Model file for the job. Use its own axes, mm. Give positions to 0.01 mm unless a question says otherwise; leave off trailing zeros. Loops run counter-clockwise (first coordinate to the right, second up) from the corner with the lowest first, then second, coordinate; pieces in that order, holes last. Notation, with made-up numbers: M 0,2 L 18,2 A12 cw 18,6 Z; hole C -38.75,-15.75 d11. An arc over 180 degrees is marked long. Answer in a Markdown table with one row per item.
```python
from build123d import *

# Parameters (mm, degrees)
SKETCH_1_W          = 46
SKETCH_1_H          = 54
EXTRUDE_1_DEPTH     = 4
SKETCH_5_R          = 1.525
CUT_EXTRUDE_1_DEPTH = 54
FILLET_1_R          = 2


with BuildPart() as part:
    # 草图1 → 凸台-拉伸1 (new body)
    with BuildSketch(Plane.XY):
        Rectangle(SKETCH_1_W, SKETCH_1_H)
    extrude(amount=EXTRUDE_1_DEPTH)

    # 草图5 → 切除-拉伸1 (cut)
    with BuildSketch(Plane(origin=(0, 0, 0), x_dir=(-1, 0, 0), z_dir=(0, 0, -1))):
        with Locations((5, -24)):
            Circle(SKETCH_5_R)
        with Locations((-15, -24)):
            Circle(SKETCH_5_R)
        with Locations((-19, 5.310310448)):
            Circle(SKETCH_5_R)
        with Locations((19, 5.310310448)):
            Circle(SKETCH_5_R)
    extrude(amount=-CUT_EXTRUDE_1_DEPTH, mode=Mode.SUBTRACT)

    # 圆角1
    fillet_1_edges = [part.edges().sort_by_distance(p)[0] for p in [
        (23, -27, 2),
        (-23, -27, 2),
        (-23, 27, 2),
        (23, 27, 2),
    ]]
    fillet(fillet_1_edges, radius=FILLET_1_R)


solid = part.part
```
(1) Wall check: L1, parallel to Y at x = 15, z = 1 (3 decimals); L2, parallel to Y at x = -19, z = 2.1; L3, parallel to X at y = 4.5, z = 1.8. Give the ranges that are in metal, low to high.
Established:
| item | result |
|---|---|
| L1 | y = -27 to -25.525, -22.475 to 27 |
| L2 | y = -27 to 3.79, 6.84 to 27 |
| L3 | x = -23 to -20.29, -17.71 to 17.71, 20.29 to 23 |
(2) Saw through at A-A, the plane y = -24. Give the cut face in (x, z) (3 decimals).
Established:
| item | result |
|---|---|
| outline | M -23,0 L -6.525,0 L -6.525,4 L -23,4 Z; M -3.475,0 L 13.475,0 L 13.475,4 L -3.475,4 Z; M 16.525,0 L 23,0 L 23,4 L 16.525,4 Z |
(3) Saw through at B-B, the plane x = 15. Give the cut face in (y, z) (3 decimals), and give its area (3 significant figures).
Established:
| item | result |
|---|---|
| outline | M -27,0 L -25.525,0 L -25.525,4 L -27,4 Z; M -22.475,0 L 27,0 L 27,4 L -22.475,4 Z |
| area | 204 mm2 |
(4) Flat gauge pin, fed straight in: P1, Ø1.8, axis at x = 15, y = -24, coming from the +Z side. Where does the tip first touch, or does it go through?
Established:
| item | result |
|---|---|
| P1 | passes through |
(5) Mould opens along Y. For faces 1 (the cylindrical face through (22.4, 26.43, 2.03)), 2 (the cylindrical face through (14.296, -25.353, 1.972)), 3 (the flat face through (0, 0, 4)) say: pulls with the +Y half, pulls with the -Y half, needs draft (parallel to the pull), parting line crosses it, or undercut.
Established:
| item | result |
|---|---|
| face 1 | pulls with the +Y half |
| face 2 | undercut |
| face 3 | needs draft |
